The listing builds one solid part. Answer for the finished solid, in the listing's coordinates (mm). A direction names the side the tool comes from. Give positions to 0.01 mm unless a question says otherwise; leave off trailing zeros. Write each loop counter-clockwise with the first axis right and the second up, starting at its lowest first coordinate (ties: lowest second). Pieces come first, ordered by that corner, then holes.
```python
from build123d import *

# Parameters (mm, degrees)
EXTRUDE_1_DEPTH     = 10
SKETCH_2_R          = 10
EXTRUDE_2_DEPTH     = 12
SKETCH_3_R          = 10
EXTRUDE_3_DEPTH     = 9
SKETCH_4_R          = 12
SKETCH_4_R_2        = 10
EXTRUDE_4_DEPTH     = 2
CHAMFER_1_SIZE      = 0.5
CHAMFER_2_SIZE      = 2
SKETCH_5_R          = 2
CUT_EXTRUDE_1_DEPTH = 6
SKETCH_6_R          = 1.3
CUT_EXTRUDE_2_DEPTH = 6
CUT_EXTRUDE_3_REACH = 76.82
SKETCH_8_W          = 28.241567454
SKETCH_8_H          = 3
CUT_EXTRUDE_4_DEPTH = 5
SKETCH_9_R          = 5
CUT_EXTRUDE_5_DEPTH = 10
SKETCH_10_R         = 5
CUT_EXTRUDE_6_DEPTH = 10
FILLET_1_SIZE       = 5


# Some blends are built 0.0001 mm under size
with BuildPart() as part:
    # 草图1 → 凸台-拉伸1 (new body)
    with BuildSketch(Plane.XY):
        with BuildLine():
            Line((57, 14), (0, 14))
            ThreePointArc((0, 14), (-14, 0), (0, -14))
            Line((0, -14), (57, -14))
            ThreePointArc((57, -14), (71, 0), (57, 14))
        make_face()
    extrude(amount=EXTRUDE_1_DEPTH)

    # 草图2 → 凸台-拉伸2 (add)
    with BuildSketch(Plane.XY.offset(10)):
        Circle(SKETCH_2_R)
    extrude(amount=EXTRUDE_2_DEPTH)

    # 草图3 → 凸台-拉伸3 (add)
    with BuildSketch(Plane(origin=(0, 0, 0), x_dir=(-1, 0, 0), z_dir=(0, 0, -1))):
        with Locations((-57, 0)):
            Circle(SKETCH_3_R)
    extrude(amount=EXTRUDE_3_DEPTH)

    # 草图4 → 凸台-拉伸4 (add)
    with BuildSketch(Plane(origin=(0, 0, 0), x_dir=(-1, 0, 0), z_dir=(0, 0, -1))):
        with Locations(Location((-57, 0, 0), (0, 0, 180))):
            Circle(SKETCH_4_R)
        with Locations((-57, 0)):
            Circle(SKETCH_4_R_2, mode=Mode.SUBTRACT)
    extrude(amount=EXTRUDE_4_DEPTH)

    # 倒角1
    chamfer_1_edges = [part.edges().sort_by_distance(p)[0] for p in [
        (-10, 0, 22),
        (67, 0, -9),
        (45, 0, -2),
    ]]
    chamfer(chamfer_1_edges, length=CHAMFER_1_SIZE)

    # 倒角2
    chamfer_2_edges = [part.edges().sort_by_distance(p)[0] for p in [
        (71, 0, 10),
        (28.5, 14, 10),
        (-14, 0, 10),
        (28.5, -14, 10),
        (-14, 0, 0),
        (28.5, 14, 0),
        (71, 0, 0),
        (28.5, -14, 0),
    ]]
    chamfer(chamfer_2_edges, length=CHAMFER_2_SIZE - 0.0001)  # a hair under: the kernel refuses the full size

    # 草图5 → 切除-拉伸1 (cut)
    with BuildSketch(Plane(origin=(0, 0, -9), x_dir=(-1, 0, 0), z_dir=(0, 0, -1))):
        with Locations((-57, 5)):
            Circle(SKETCH_5_R)
        with Locations((-52.669872981, -2.5)):
            Circle(SKETCH_5_R)
        with Locations((-61.330127019, -2.5)):
            Circle(SKETCH_5_R)
    extrude(amount=-CUT_EXTRUDE_1_DEPTH, mode=Mode.SUBTRACT)

    # 草图6 → 切除-拉伸2 (cut)
    with BuildSketch(Plane.XY.offset(22)):
        with Locations((0, 7)):
            Circle(SKETCH_6_R)
        with Locations((7, 0)):
            Circle(SKETCH_6_R)
        with Locations((0, -7)):
            Circle(SKETCH_6_R)
        with Locations((-7, 0)):
            Circle(SKETCH_6_R)
    extrude(amount=-CUT_EXTRUDE_2_DEPTH, mode=Mode.SUBTRACT)

    # 草图7 → 切除-拉伸3 (cut, up to next)
    with BuildSketch(Plane.XY.offset(10), mode=Mode.PRIVATE) as cut_extrude_3_sk1:
        with BuildLine():
            ThreePointArc((41.508066615, -7), (40, 0), (41.508066615, 7))
            Line((41.508066615, 7), (13.266499161, 7))
            ThreePointArc((13.266499161, 7), (14.560176637, 3.605725487), (15, 0))
            ThreePointArc((15, 0), (14.560176637, -3.605725487), (13.266499161, -7))
            Line((13.266499161, -7), (41.508066615, -7))
        make_face()
    cut_extrude_3_tool1 = extrude(cut_extrude_3_sk1.sketch, amount=-CUT_EXTRUDE_3_REACH, mode=Mode.PRIVATE) & part.part
    add(cut_extrude_3_tool1.solids().sort_by_distance((27.463612, 0, 10))[0], mode=Mode.SUBTRACT)

    # 草图8 → 切除-拉伸4 (cut)
    with BuildSketch(Plane(origin=(0, 0, 0), x_dir=(-1, 0, 0), z_dir=(0, 0, -1))):
        with Locations((-27.387282888, 8.5)):
            Rectangle(SKETCH_8_W, SKETCH_8_H)
        with Locations((-27.387282888, -8.5)):
            Rectangle(SKETCH_8_W, SKETCH_8_H)
    extrude(amount=-CUT_EXTRUDE_4_DEPTH, mode=Mode.SUBTRACT)

    # 草图9 → 切除-拉伸5 (cut)
    with BuildSketch(Plane.XY.offset(10)):
        with Locations((57, 0)):
            Circle(SKETCH_9_R)
    extrude(amount=-CUT_EXTRUDE_5_DEPTH, mode=Mode.SUBTRACT)

    # 草图10 → 切除-拉伸6 (cut)
    with BuildSketch(Plane(origin=(0, 0, 0), x_dir=(-1, 0, 0), z_dir=(0, 0, -1))):
        Circle(SKETCH_10_R)
    extrude(amount=-CUT_EXTRUDE_6_DEPTH, mode=Mode.SUBTRACT)

    # 圆角1
    # a fillet whose section is not a circle: 5 mm, written as the material it takes off along each edge
    with BuildSketch(Plane(origin=(57, 0, 10), x_dir=(1, 0, 0), z_dir=(0, -1, 0))) as fillet_1_piece_1:
        with BuildLine():
            add(Edge.make_bspline([(5 + FILLET_1_SIZE, 0), (5 + FILLET_1_SIZE * 0.831801948466, 0), (5 + FILLET_1_SIZE * 0.663603896932, 0), (5 + FILLET_1_SIZE * 0.292893218813, -FILLET_1_SIZE * 0.0716919198361), (5 + FILLET_1_SIZE * 0.0716919198361, -FILLET_1_SIZE * 0.292893218813), (5, -FILLET_1_SIZE * 0.663603896932), (5, -FILLET_1_SIZE * 0.831801948466), (5, -FILLET_1_SIZE)], knots=[0, 0, 0, 0, 0, 0, 0.5, 0.5, 1, 1, 1, 1, 1, 1], degree=5))
            Line((5, -FILLET_1_SIZE), (5, 0))
            Line((5, 0), (5 + FILLET_1_SIZE, 0))
        make_face()
    revolve(axis=Axis((57, 0, 10), (0, 0, 1)), mode=Mode.SUBTRACT)
    with BuildSketch(Plane(origin=(0, 0, 0), x_dir=(-1, 0, 0), z_dir=(0, -1, 0))) as fillet_1_piece_2:
        with BuildLine():
            add(Edge.make_bspline([(5 + FILLET_1_SIZE, 0), (5 + FILLET_1_SIZE * 0.831801948466, 0), (5 + FILLET_1_SIZE * 0.663603896932, 0), (5 + FILLET_1_SIZE * 0.292893218813, -FILLET_1_SIZE * 0.0716919198361), (5 + FILLET_1_SIZE * 0.0716919198361, -FILLET_1_SIZE * 0.292893218813), (5, -FILLET_1_SIZE * 0.663603896932), (5, -FILLET_1_SIZE * 0.831801948466), (5, -FILLET_1_SIZE)], knots=[0, 0, 0, 0, 0, 0, 0.5, 0.5, 1, 1, 1, 1, 1, 1], degree=5))
            Line((5, -FILLET_1_SIZE), (5, 0))
            Line((5, 0), (5 + FILLET_1_SIZE, 0))
        make_face()
    revolve(axis=Axis((0, 0, 0), (0, 0, -1)), mode=Mode.SUBTRACT)


solid = part.part
```
Item 1: A cutting plane is placed at A-A, the plane x = 16. Give the vertices of the cut face in (y, z), plus the area to 3 significant figures.
Conclusion:
outline: (-14, 2) - (-12, 0) - (-10, 0) - (-10, 5) - (-7, 5) - (-7, 10) - (-12, 10) - (-14, 8) - close; (7, 5) - (10, 5) - (10, 0) - (12, 0) - (14, 2) - (14, 8) - (12, 10) - (7, 10) - close
area: 102 mm2
Item 2: Determine the mould class of faces 4 (the face through (45.01, -0.53, -0.74)), 5 (the face through (28, 8, 10)), 6 (the face through (7, 0, 16)), 7 (the face through (29, 13, 1)) for opening direction Y: pulls with the +Y half, pulls with the -Y half, needs draft (parallel to the pull), parting line crosses it, or undercut.
Conclusion:
face 4: parting line crosses it
face 5: needs draft
face 6: undercut
face 7: pulls with the +Y half
Item 3: Each of these flat-tipped pins is pushed along its axis until it touches: P1, Ø3, axis at x = 7, y = 0, coming from the -Z side; P2, Ø2, axis at x = 62, y = -3, coming from the -Z side; P3, Ø12, axis at x = 4, y = -9.5, coming from the -Z side. Where does it stop, or does it pass through?
Conclusion:
P1: stops at z = 0.07
P2: stops at z = -3
P3: stops at z = 0
Item 4: A cutting plane is placed at C-C, the plane z = 15. Give the vertices of the cut face in (x, y).
Conclusion:
outline: circle Ø20 at (0, 0)
Item 5: Consider probe 1 along Y at (x, z) = (0, 19); probe 2 along Y at (x, z) = (0, 7); probe 3 along Z at (x, y) = (8.5, -3.75). Determine where each line is inside the solid, lowest interval first.
Conclusion:
probe 1: y = -10 to -8.3, -5.7 to 5.7, 8.3 to 10
probe 2: y = -14 to -5, 5 to 14
probe 3: z = 0.01 to 22
Item 6: A cutting plane is placed at D-D, the plane z = 6.5. Count the separate pieces of the cut face and the enclosed holes in it, plus the area to 3 significant figures.
Conclusion:
separate pieces: 1
enclosed holes: 3
area: 1,690 mm2
Item 7: A cutting plane is placed at B-B, the plane z = 19. Give the vertices of the cut face in (x, y), plus the area to 3 significant figures.
Conclusion:
outline: circle Ø20 at (0, 0); hole circle Ø2.6 at (-7, 0); hole circle Ø2.6 at (0, -7); hole circle Ø2.6 at (0, 7); hole circle Ø2.6 at (7, 0)
area: 293 mm2
Item 8: Which of the six approach directions +Z, -Z, +X, -X, +Y, -Y give full straight-line access (tool end or side, diameter ignored) to faces 1 (the face through (-0.28, -8.27, 19.04)), 2 (the face through (-12.122, 0.267, 0.125)), 3 (the face through (48, -5, -2))?
Conclusion:
face 1: +Z
face 2: -Z, -X
face 3: -Z
